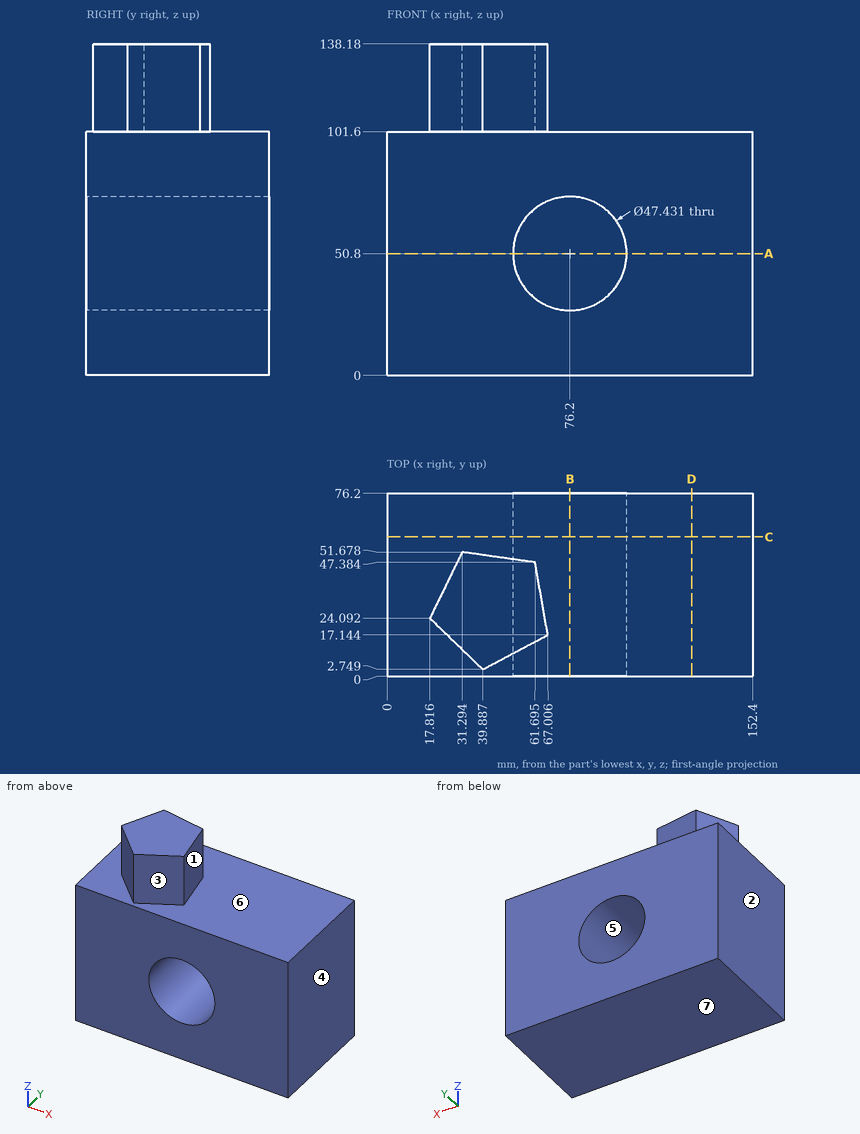
Design review of the part shown in the three views and the two pictorial views. Dimensions are in mm from the part's minimum x, y and z. A direction names the side the tool comes from. Give positions to 0.01 mm unless a question says otherwise; leave off trailing zeros. Loops run counter-clockwise (first coordinate to the right, second up) from the corner with the lowest first, then second, coordinate; pieces in that order, holes last. Notation, with made-up numbers: (48, 16.25) - (58, 16.25) arc R22 cw to (58, 38.25) - close; hole circle Ø5 at (-34, 29.5). An arc over 180 degrees is marked (long way). Use CSV: the item, a comma, the result in double quotes. Start each with the question number.
1. Add section D-D (x = 127). State the section outline as (y, z) points.
2. Wall thickness on L1, parallel to Z at x = 76, y = 58 (1 decimal); L2, parallel to X at y = 48, z = 50; L3, parallel to X at y = 38, z = 47: over which ranges is each line inside the solid? List them lowest first.
3. Add section B-B (x = 76.2). State the section outline as (y, z) points (1 decimal).
4. Add section A-A (z = 50.8). State the section outline as (x, y) points (1 decimal), plus the area to 3 significant figures.
5. Draft analysis for pull direction Z (two halves, no side actions). For the marked faces 4, 5, 6 and 7, state which applies: released by +Z, released by -Z, zero draft, split by the parting line, or undercut.
6. Add section C-C (y = 58). State the section outline as (x, z) points (1 decimal).
7. Machinability: for the marked faces 1, 2 and 3, which of the approach directions +Z, -Z, +X, -X, +Y, -Y give a long, thin tool a straight path to every point of the face, cutting with its end or side? Answer none if there is none.
Results found:
1,outline,"(0, 0) - (76.2, 0) - (76.2, 101.6) - (0, 101.6) - close"
2,L1,"z = 0 to 27.1, 74.5 to 101.6"
2,L2,"x = 0 to 52.5, 99.9 to 152.4"
2,L3,"x = 0 to 52.79, 99.61 to 152.4"
3,outline,"(0, 0) - (76.2, 0) - (76.2, 27.1) - (0, 27.1) - close; (0, 74.5) - (76.2, 74.5) - (76.2, 101.6) - (0, 101.6) - close"
4,outline,"(0, 0) - (52.5, 0) - (52.5, 76.2) - (0, 76.2) - close; (99.9, 0) - (152.4, 0) - (152.4, 76.2) - (99.9, 76.2) - close"
4,area,"8,000 mm²"
5,face 4,"zero draft"
5,face 5,"undercut"
5,face 6,"released by +Z"
5,face 7,"released by -Z"
6,outline,"(0, 0) - (152.4, 0) - (152.4, 101.6) - (0, 101.6) - close; hole circle Ø47.4 at (76.2, 50.8)"
7,face 1,"+Z, +X, +Y"
7,face 2,"+Z, -Z, -X, +Y, -Y"
7,face 3,"+Z, +X, -Y"
